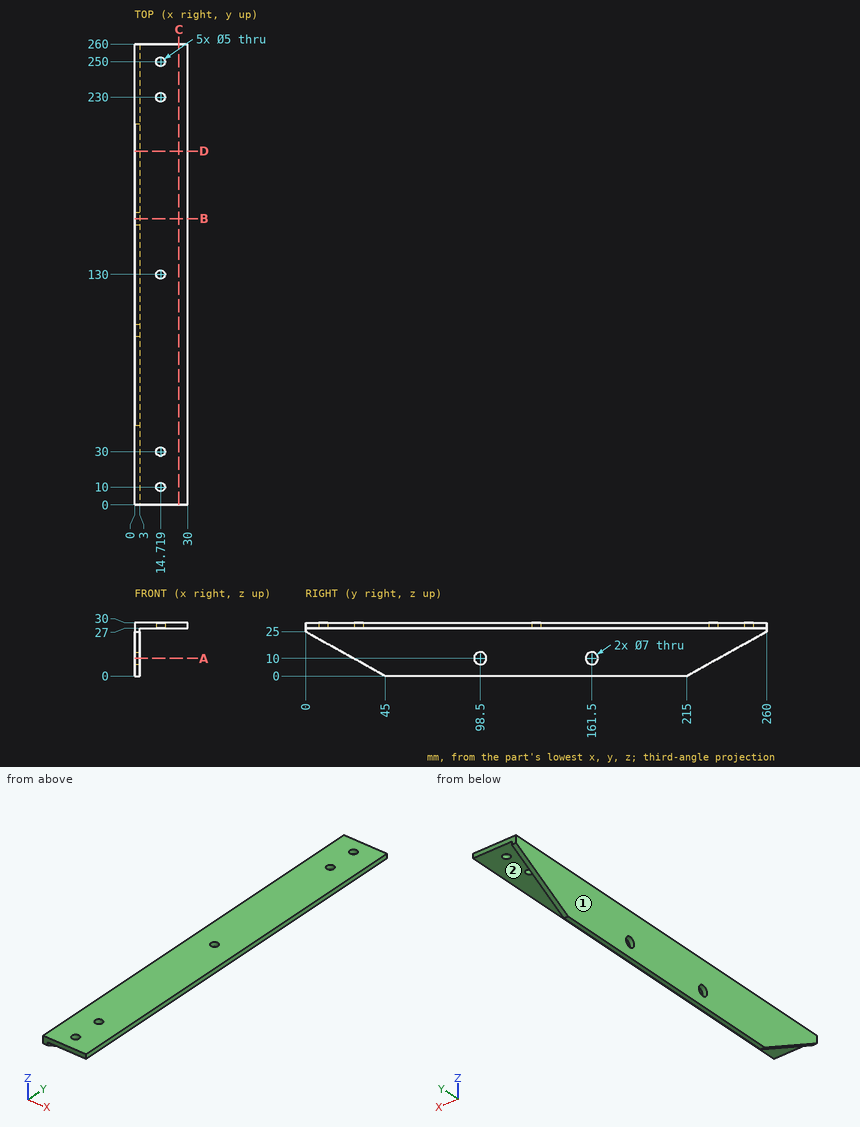
Study the drawing (mm; zero at the part's minimum x, y, z) and answer. A direction names the side the tool comes from. Give positions to 0.01 mm unless a question says otherwise; leave off trailing zeros. Write each loop counter-clockwise with the first axis right and the second up, starting at its lowest first coordinate (ties: lowest second). Pieces come first, ordered by that corner, then holes. Notation, with made-up numbers: (-30, 78) -> (-9, 78) arc R23 cw to (-9, 112) -> close; hole circle Ø3 at (39, -34.75). An arc over 180 degrees is marked (long way). Answer as a JSON object with one key per item and string values. Group by question number.
1) A tool of negligible diameter and unlimited length cuts with its end or side. For the marked faces 1 and 2, from which of +Z, -Z, +X, -X, +Y, -Y can it reach the whole face along a straight path? Write none if from no direction.
2) Find section C-C (x = 25). Write down the section's boundary in (y, z).
3) Find section B-B (y = 161.5). Write down the section's boundary in (x, z), and give its area (3 significant figures).
4) Consider L1, parallel to X at y = 230, z = 27.95; L2, parallel to Z at x = 1.2, y = 98.5; L3, parallel to Z at x = 5.5, y = 203. Determine where each line is inside the solid, lowest interval first. Write a range as from..to.
5) Find section A-A (z = 10). Write down the section's boundary in (x, y), and give its area (3 significant figures).
6) Find section D-D (y = 199.5). Write down the section's boundary in (x, z), and give its area (3 significant figures).
7) Each of these flat-tipped pins is pushed along its axis until it touches: P1, Ø8, axis at x = 8.5, z = 6, coming from the +Y side; P2, Ø5, axis at x = 12, y = 32.5, coming from the -Z side; P3, Ø12, axis at x = 4, z = 8.5, coming from the +Y side; P4, Ø1.5, axis at y = 137.5, z = 25, coming from the +X side. Where does it stop, or does it pass through?
Values follow:
{
 "1": {"face 1": "+Z, -Z, -X, +Y, -Y", "face 2": "-Z, +X, +Y, -Y"},
 "2": {"outline": "(0, 27) -> (260, 27) -> (260, 30) -> (0, 30) -> close"},
 "3": {"outline": "(0, 0) -> (3, 0) -> (3, 6.5) -> (0, 6.5) -> close; (0, 13.5) -> (3, 13.5) -> (3, 27) -> (30, 27) -> (30, 30) -> (0, 30) -> close", "area": "150 mm2"},
 "4": {"L1": "x = 0..12.22, 17.22..30", "L2": "z = 0..6.5, 13.5..30", "L3": "z = 27..30"},
 "5": {"outline": "(0, 27) -> (3, 27) -> (3, 95) -> (0, 95) -> close; (0, 102) -> (3, 102) -> (3, 158) -> (0, 158) -> close; (0, 165) -> (3, 165) -> (3, 233) -> (0, 233) -> close", "area": "576 mm2"},
 "6": {"outline": "(0, 0) -> (3, 0) -> (3, 27) -> (30, 27) -> (30, 30) -> (0, 30) -> close", "area": "171 mm2"},
 "7": {"P1": "passes through", "P2": "stops at z = 27", "P3": "stops at y = 240.95", "P4": "stops at x = 3"}
}
